The figure shows three views and two pictorial views of one solid part (mm, origin at its lowest corner). Answer the questions. Coordinates: 2 decimals unless noted, no trailing zeros. Write each loop counter-clockwise with the first axis right and the second up, starting at its lowest first coordinate (ties: lowest second). Pieces come first, ordered by that corner, then holes. Notation, with made-up numbers: M -9.5,60 L 26.5,60 A15 ccw 26.5,86 Z; hole C -39,82 d6. An arc over 180 degrees is marked long. Write item = value, one per line.
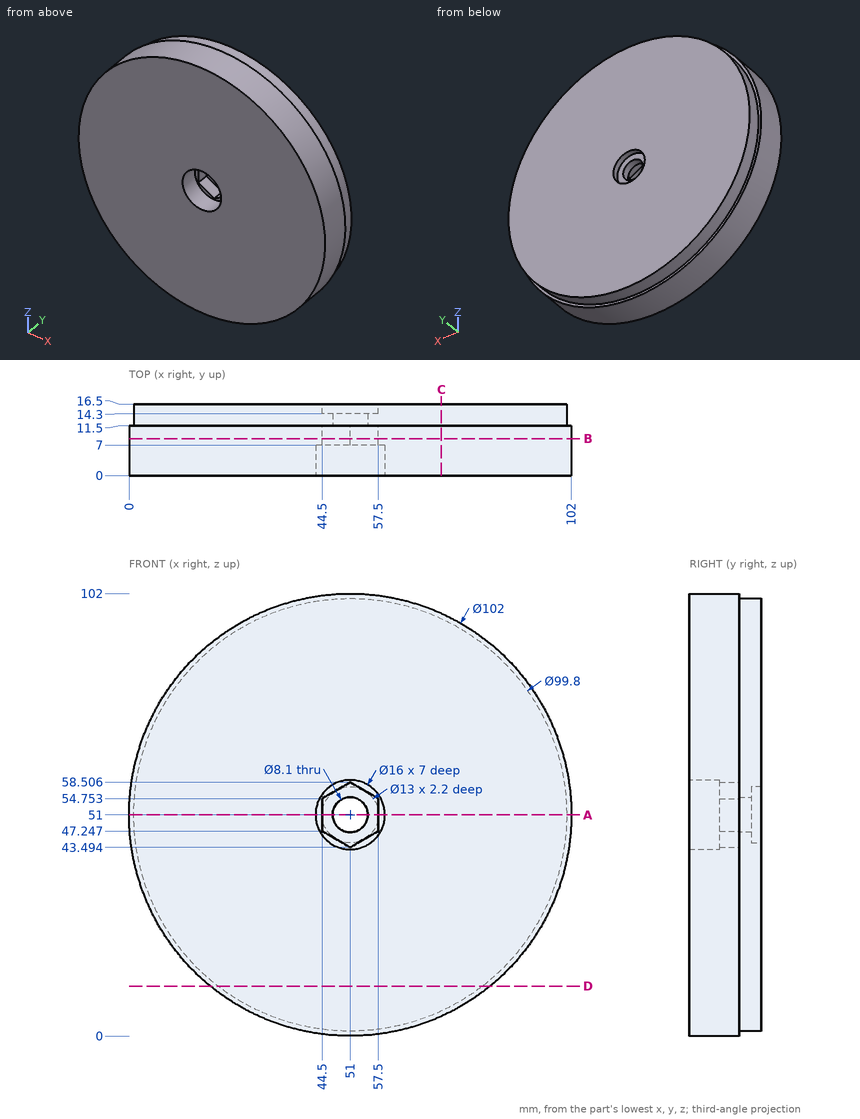
Item 1: Find section C-C (x = 72). Determine the outline of the cut face in (y, z) (1 decimal), and give its area (3 significant figures).
Worked answers:
outline = M 0,4.5 L 11.5,4.5 L 11.5,5.7 L 16.5,5.7 L 16.5,96.3 L 11.5,96.3 L 11.5,97.5 L 0,97.5 Z
area = 1,520 mm²
Item 2: Find section A-A (z = 51). Determine the outline of the cut face in (x, y), and give its area (3 significant figures).
Worked answers:
outline = M 0,0 L 43,0 L 43,7 L 44.5,7 L 44.5,11.5 L 46.95,11.5 L 46.95,14.3 L 44.5,14.3 L 44.5,16.5 L 1.1,16.5 L 1.1,11.5 L 0,11.5 Z; M 55.05,11.5 L 57.5,11.5 L 57.5,7 L 59,7 L 59,0 L 102,0 L 102,11.5 L 100.9,11.5 L 100.9,16.5 L 57.5,16.5 L 57.5,14.3 L 55.05,14.3 Z
area = 1,450 mm²
Item 3: Flat-ended cylindrical pins translate along their axes: pin 1 (8 mm diameter, centred on x = 19.5, z = 11, fed in from +Y); pin 2 (5 mm diameter, centred on y = 14.5, z = 49.5, fed in from -X); pin 3 (10.5 mm diameter, centred on x = 51, z = 51, fed in from +Y); pin 4 (2 mm diameter, centred on x = 22, y = 7.5, fed in from +Z) (1 decimal). Find the tip coordinate at first contact, or state that the pin passes through.
Worked answers:
pin_1 = 16.5
pin_2 = 1.1
pin_3 = 14.3
pin_4 = 93.6
Item 4: Consider line 1 along X through (y, z) = (14.8, 51); line 2 along X through (y, z) = (3.75, 51); line 3 along Z through (x, y) = (52.5, 5.25). Determine where each line is inside the solid, lowest interval first. Write a range as from..to.
Worked answers:
line_1 = 1.1..44.5, 57.5..100.9
line_2 = 0..43, 59..102
line_3 = 0.02..43.14, 58.86..101.98
Item 5: Find section B-B (y = 8.5). Determine the outline of the cut face in (x, z) (1 decimal), and give its area (4 significant figures).
Worked answers:
outline = C 51,51 d102; hole M 44.5,47.2 L 51,43.5 L 57.5,47.2 L 57.5,54.8 L 51,58.5 L 44.5,54.8 Z
area = 8,025 mm²
Item 6: Find section D-D (z = 11.5). Determine the outline of the cut face in (x, y).
Worked answers:
outline = M 18.74,0 L 83.26,0 L 83.26,11.5 L 81.49,11.5 L 81.49,16.5 L 20.51,16.5 L 20.51,11.5 L 18.74,11.5 Z
